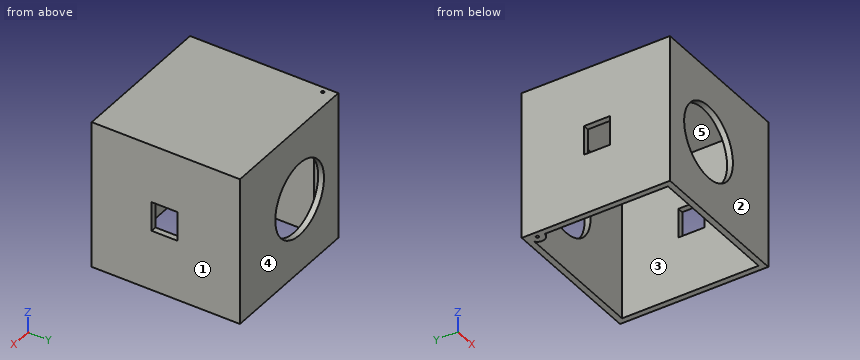
```python
from build123d import *

# Parameters (mm, degrees)
F0_W     = 254
F0_H     = 254
F1_DEPTH = 254
F3_D     = 5
F4_T     = -10
F5_R     = 62.949933
F6_DEPTH = 254.001
F7_W     = 44.732734
F7_H     = 50.324321
F8_DEPTH = 254.001


with BuildPart() as f1:
    # F0 (on Front) → F1 (new body)
    with BuildSketch(Plane.XZ):
        with Locations((127, 127)):
            Rectangle(F0_W, F0_H)
    extrude(amount=F1_DEPTH)

    # F3 (through all)
    with Locations(Plane.XY.offset(254)):
        with Locations((10, -20)):
            Hole(F3_D / 2)

    # F4
    f4_openings = [f1.faces().sort_by_distance(p)[0] for p in [
        (127.035619, -127.032575, 0),
    ]]
    offset(amount=F4_T, openings=f4_openings)

    # F5 (on face) → F6 (cut, through all)
    with BuildSketch(Plane.XZ.offset(254)):
        with Locations((99.736825, 127.332494)):
            Circle(F5_R)
    extrude(amount=-F6_DEPTH, mode=Mode.SUBTRACT)

    # F7 (on face) → F8 (cut, through all)
    with BuildSketch(Plane.YZ.offset(254)):
        with Locations((-129.031144, 128.951653)):
            Rectangle(F7_W, F7_H)
    extrude(amount=-F8_DEPTH, mode=Mode.SUBTRACT)


solid = f1.part
```
The listing builds one solid part. Answer for the finished solid, in the listing's coordinates (mm). Face numbers are marked on the shaded views. A direction names the side the tool comes from. Coordinates: 2 decimals unless noted, no trailing zeros. Write each loop counter-clockwise with the first axis right and the second up, starting at its lowest first coordinate (ties: lowest second). Pieces come first, ordered by that corner, then holes. Notation, with made-up numbers: (-12.5, 23) - (24.5, 23) arc R15 cw to (24.5, 52) - close; hole circle Ø7 at (34, 49). An arc over 180 degrees is marked (long way). One line per item, written item: value.
1) Find section D-D (x = 226). Give the vertices of the cut face in (y, z), and give its area (3 significant figures).
Geometry check:
outline: (-254, 0) - (-244, 0) - (-244, 244) - (-10, 244) - (-10, 0) - (0, 0) - (0, 254) - (-254, 254) - close
area: 7,420 mm2
2) A tool of negligible diameter and unlimited length cuts with its end or side. For the marked faces 4 and 5, from which of +Z, -Z, +X, -X, +Y, -Y can it reach the whole face along a straight path? Write none if from no direction.
Geometry check:
face 4: +Z, -Z, +X, -X, +Y
face 5: -Z
3) Find section C-C (z = 86). Give the vertices of the cut face in (x, y).
Geometry check:
outline: (0, -254) - (52.26, -254) - (52.26, -244) - (10, -244) - (10, -32.5) arc R12.5 ccw to (17.5, -10) - (52.26, -10) - (52.26, 0) - (0, 0) - close; (147.22, -254) - (254, -254) - (254, 0) - (147.22, 0) - (147.22, -10) - (244, -10) - (244, -244) - (147.22, -244) - close; hole circle Ø5 at (10, -20)
4) Consider line 1 along Y through (x, z) = (204, 66); line 2 along X through (y, z) = (-88, 209); line 3 along Z through (x, y) = (103.5, -57). Determine where each line is inside the solid, lowest interval first. Write a range as from..to.
Geometry check:
line 1: y = -254..-244, -10..0
line 2: x = 0..10, 244..254
line 3: z = 244..254
5) Find section A-A (y = -118.5). Give the vertices of the cut face in (x, z).
Geometry check:
outline: (0, 0) - (10, 0) - (10, 103.79) - (0, 103.79) - close; (0, 154.11) - (10, 154.11) - (10, 244) - (244, 244) - (244, 154.11) - (254, 154.11) - (254, 254) - (0, 254) - close; (244, 0) - (254, 0) - (254, 103.79) - (244, 103.79) - close
6) For a pull along Y with two mould halves and no side action, classify the marked faces 1, 2 and 3 as pulls with the +Y half, pulls with the -Y half, needs draft (parallel to the pull), parting line crosses it, or undercut.
Geometry check:
face 1: needs draft
face 2: pulls with the -Y half
face 3: undercut
7) Find section B-B (z = 140.5). Give the vertices of the cut face in (x, y).
Geometry check:
outline: (0, -254) - (38.18, -254) - (38.18, -244) - (10, -244) - (10, -151.4) - (0, -151.4) - close; (0, -106.66) - (10, -106.66) - (10, -32.5) arc R12.5 ccw to (17.5, -10) - (38.18, -10) - (38.18, 0) - (0, 0) - close; (161.29, -254) - (254, -254) - (254, -151.4) - (244, -151.4) - (244, -244) - (161.29, -244) - close; (161.29, -10) - (244, -10) - (244, -106.66) - (254, -106.66) - (254, 0) - (161.29, 0) - close; hole circle Ø5 at (10, -20)
